Autodesk Inventor part; units mm, degrees
ref_plane "YZ Plane" through (0, 0, 0) normal (1, 0, 0) x (0, 1, 0)
ref_plane "XZ Plane" through (0, 0, 0) normal (0, 1, 0) x (-1, 0, 0)
ref_plane "XY Plane" through (0, 0, 0) normal (0, 0, 1) x (1, 0, 0)
sketch "Sketch1" plane through (0, 0, 0) normal (0, 1, 0) x (-1, 0, 0)
  line L0 (31.75, 19) -> (-31.75, 19)
  line L1 (-31.75, 19) -> (-31.75, -19)
  line L2 (-31.75, -19) -> (31.75, -19)
  line L3 (31.75, -19) -> (31.75, 19)
  line L4 (31.75, 19) -> (31.75, 14) construction
  line L5 (31.75, 14) -> (31.75, -14) construction
  line L6 (31.75, 19) -> (25.5, 19) construction
  line L7 (25.5, 19) -> (8.5, 19) construction
  line L8 (8.5, 19) -> (-8.5, 19) construction
  line L9 (-8.5, 19) -> (-25.5, 19) construction
  line L10 (31.75, 14) -> (-25.5, 14) construction
  line L11 (-25.5, 14) -> (-25.5, -14) construction
  line L12 (-25.5, -14) -> (-8.5, -14) construction
  line L13 (-8.5, -14) -> (8.5, -14) construction
  line L14 (8.5, -14) -> (25.5, -14) construction
  line L15 (25.5, -14) -> (31.75, -14) construction
  line L16 (25.5, 14) -> (25.5, -14) construction
  line L17 (8.5, 14) -> (8.5, -14) construction
  line L18 (-8.5, 14) -> (-8.5, -14) construction
  circle A0 centre (25.5, 14) radius 2.25
  circle A1 centre (25.5, -14) radius 2.25
  circle A2 centre (8.5, -14) radius 2.25
  circle A3 centre (-8.5, -14) radius 2.25
  circle A4 centre (-25.5, -14) radius 2.25
  circle A5 centre (-25.5, 14) radius 2.25
  circle A6 centre (-8.5, 14) radius 2.25
  circle A7 centre (8.5, 14) radius 2.25
  point P0 (0, 0)
  dimension "d0" = 63.5
  dimension "d1" = 38
  dimension "d5" = 17
  dimension "d6" = 17
  dimension "d7" = 17
extrude "Extrusion1" add sketch "Sketch1" along normal blind 17
sketch "Sketch2" plane through (0, 17, 0) normal (0, 1, 0) x (1, 0, 0)
  line L0 (-16.5, -9.75) -> (16.5, -9.75)
  line L1 (16.5, -9.75) -> (16.5, 9.75)
  line L2 (16.5, 9.75) -> (-16.5, 9.75)
  line L3 (-16.5, 9.75) -> (-16.5, -9.75)
  line L4 (-16.5, -9.75) -> (16.5, 9.75) construction
  line L5 (16.5, -9.75) -> (-16.5, 9.75) construction
  point P0 (0, 0)
  dimension "d12" = 33
  dimension "d13" = 19.5
extrude "Extrusion2" cut sketch "Sketch2" against normal through all
sketch "Sketch3" plane through (-31.75, 0, -19) normal (-1, 0, 0) x (0, 0, 1)
  line L0 (19, 0) -> (19, 17) construction
  line L1 (38, 17) -> (0, 17) construction
  line L2 (0, 0) -> (0, 17) construction
  line L3 (0, 8.5) -> (38, 8.5) construction
  line L4 (38, 0) -> (38, 17) construction
  circle A0 centre (19, 8.5) radius 2.08 construction
hole "Hole1" at (-31.75, 8.5, 0) direction (1, 0, 0) diameter 10 depth 8.6 tip angle 118
sketch "Sketch4" plane through (-16.5, 17, 9.75) normal (1, 0, 0) x (0, 0, -1)
  line L0 (-9.25, -17) -> (-9.25, 0) construction
  line L1 (-9.25, -8.5) -> (28.75, -8.5) construction
  line L2 (28.75, -17) -> (28.75, 0) construction
  circle A0 centre (9.75, -8.5) radius 2.55
  point P0 (9.75, -17)
  dimension "d23" = 5.1
extrude "Extrusion3" cut sketch "Sketch4" against normal through all
sketch "Sketch5" plane through (-31.75, 0, 19) normal (0, 0, 1) x (1, 0, 0)
  line L0 (63.5, 0) -> (63.5, 17) construction
  line L1 (63.5, 8.5) -> (48.8, 8.5) construction
  circle A0 centre (48.8, 8.5) radius 5
  point P0 (31.75, 0)
  dimension "d26" = 14.7
  dimension "d27" = 10
extrude "Extrusion4" cut sketch "Sketch5" against normal blind 10
sketch "Sketch6" plane through (-31.75, 0, 19) normal (0, 0, 1) x (1, 0, 0)
  line L0 (63.5, 0) -> (63.5, 17) construction
  line L1 (63.5, 8.5) -> (48.8, 8.5) construction
  point P0 (31.75, 0)
  dimension "d30" = 14.7
hole "Hole2" at (17.05, 8.5, 19) direction (0, 0, -1) diameter 9.5 depth 17 tip angle 118
properties part number "Distributore"
The listing builds one solid part. Answer for the finished solid, in the listing's coordinates (mm). A direction names the side the tool comes from. Round coordinates to 2 decimals unless told otherwise and drop trailing zeros. Order: outer loops, then holes, each group sorted by start corner. A loop starts at its lowest first (then second) coordinate and runs counter-clockwise, first axis right, second up. Notation, with made-up numbers: (62, 89) -> (110, 89) arc R17 ccw to (110, 118) -> close; hole circle Ø6 at (49.5, -2). An arc over 180 degrees is marked (long way). Answer as CSV lines item,"result".
Q1. A cutting plane is placed at C-C on x = 25.5. Determine the outline of the cut face in (y, z).
Computed values:
outline,"(0, -19) -> (17, -19) -> (17, -16.25) -> (0, -16.25) -> close; (0, -11.75) -> (17, -11.75) -> (17, 11.75) -> (0, 11.75) -> close; (0, 16.25) -> (17, 16.25) -> (17, 19) -> (0, 19) -> close"
Q2. A cutting plane is placed at D-D on z = 14. Determine the outline of the cut face in (x, y).
Computed values:
outline,"(-31.75, 0) -> (-27.75, 0) -> (-27.75, 17) -> (-31.75, 17) -> close; (-23.25, 0) -> (-10.75, 0) -> (-10.75, 17) -> (-23.25, 17) -> close; (-6.25, 0) -> (6.25, 0) -> (6.25, 17) -> (-6.25, 17) -> close; (10.75, 0) -> (23.25, 0) -> (23.25, 17) -> (10.75, 17) -> close; (27.75, 0) -> (31.75, 0) -> (31.75, 17) -> (27.75, 17) -> close; hole circle Ø10 at (17.05, 8.5)"
Q3. A cutting plane is placed at B-B on x = 0. Determine the outline of the cut face in (y, z).
Computed values:
outline,"(0, -19) -> (17, -19) -> (17, -9.75) -> (0, -9.75) -> close; (0, 9.75) -> (17, 9.75) -> (17, 19) -> (0, 19) -> close"
Q4. Given pin 1 (3 mm diameter, centred on x = 18, y = 6, fed in from +Z); pin 2 (8 mm diameter, centred on y = 8.5, z = 0, fed in from -X), each flat-ended and moving along its own axis, determine where each tip first touches the part or whether it passes through.
Computed values:
pin 1,"stops at z = 1.65"
pin 2,"stops at x = -22.55"
Q5. Which of the six approach directions +Z, -Z, +X, -X, +Y, -Y give full straight-line access (tool end or side, diameter ignored) to faces 1 (the flat face through (-31.75, 5, -4)), 2 (the flat face through (0, 9, 9.75)), 3 (the cylindrical face through (21.82, 10, 14.07))?
Computed values:
face 1,"+Z, -Z, -X, +Y, -Y"
face 2,"+Y, -Y"
face 3,"+Z"
Q6. A cutting plane is placed at A-A on z = -14. Determine the outline of the cut face in (x, y).
Computed values:
outline,"(-31.75, 0) -> (-27.75, 0) -> (-27.75, 17) -> (-31.75, 17) -> close; (-23.25, 0) -> (-10.75, 0) -> (-10.75, 17) -> (-23.25, 17) -> close; (-6.25, 0) -> (6.25, 0) -> (6.25, 17) -> (-6.25, 17) -> close; (10.75, 0) -> (23.25, 0) -> (23.25, 17) -> (10.75, 17) -> close; (27.75, 0) -> (31.75, 0) -> (31.75, 17) -> (27.75, 17) -> close"
Q7. For a pull along Y with two mould halves and no side action, classify faces 4 (the flat face through (0, 0, -12)), 5 (the cylindrical face through (-27.39, 3.543, -0.651)), 6 (the cylindrical face through (-6.714, 8.381, -12.631)), 7 (the conical face through (18.39, 8.68, -0.04)) as +Y half, -Y half, draft (parallel to the pull), parting line (faces both ways), or undercut.
Computed values:
face 4,"-Y half"
face 5,"undercut"
face 6,"draft"
face 7,"undercut"
Q8. Consider line 1 (Z direction, x = -8.5, y = 11); line 2 (Z direction, x = 1, y = 12.75); line 3 (Y direction, x = 17.05, z = 6.25). Determine where each line is inside the solid, lowest interval first. Write a range as from..to.
Computed values:
line 1,"z = -19..-16.25, -11.75..-9.75, 9.75..11.75, 16.25..19"
line 2,"z = -19..-9.75, 9.75..19"
line 3,"y = 0..3.75, 13.25..17"
